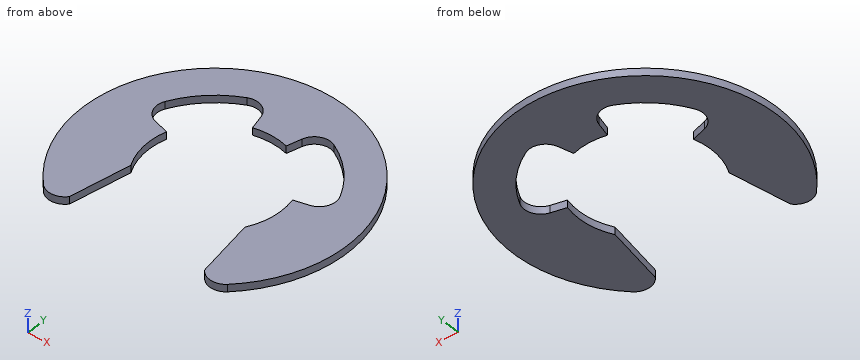
Autodesk Inventor part; units mm, degrees
ref_plane "YZ Plane" through (0, 0, 0) normal (1, 0, 0) x (0, 1, 0)
ref_plane "XZ Plane" through (0, 0, 0) normal (0, 1, 0) x (-1, 0, 0)
ref_plane "XY Plane" through (0, 0, 0) normal (0, 0, 1) x (1, 0, 0)
sketch "Sketch1" plane through (0, 0, 0) normal (0, 0, 1) x (1, 0, 0)
  arc A0 (11.7245, -15.68) -> (15.9849, -15.9849) centre (13.9867, -13.9867) ccw
  arc A1 (15.9849, -15.9849) -> (-15.9849, -15.9849) centre (0, 0) ccw
  arc A2 (-15.9849, -15.9849) -> (-11.7245, -15.68) centre (-13.9867, -13.9867) ccw
  line L0 (-11.7245, -15.68) -> (-9.8901, -5.472)
  arc A3 (-10.9218, 2.9106) -> (-9.8901, -5.472) centre (0, 0) ccw
  line L1 (-10.9218, 2.9106) -> (-13.3802, 3.5657)
  arc A4 (-15.1786, 7.5542) -> (-13.3802, 3.5657) centre (-12.6488, 6.2952) ccw
  arc A5 (-7.5542, 15.1786) -> (-15.1786, 7.5542) centre (0, 0) ccw
  arc A6 (-3.5657, 13.3802) -> (-7.5542, 15.1786) centre (-6.2952, 12.6488) ccw
  line L2 (-3.5657, 13.3802) -> (-2.9254, 10.9179)
  arc A7 (2.9254, 10.9179) -> (-2.9254, 10.9179) centre (0, 0) ccw
  line L3 (2.9254, 10.9179) -> (3.5657, 13.3802)
  arc A8 (7.5542, 15.1786) -> (3.5657, 13.3802) centre (6.2952, 12.6488) ccw
  arc A9 (15.1786, 7.5542) -> (7.5542, 15.1786) centre (0, 0) ccw
  arc A10 (13.3802, 3.5657) -> (15.1786, 7.5542) centre (12.6488, 6.2952) ccw
  line L4 (13.3802, 3.5657) -> (10.9218, 2.9106)
  arc A11 (9.8901, -5.472) -> (10.9218, 2.9106) centre (0, 0) ccw
  line L5 (9.8901, -5.472) -> (11.7245, -15.68)
  dimension "d0" = 22.606
  dimension "d2" = 11.303
extrude "Extrusion1" add sketch "Sketch1" against normal blind 1.27
properties part number "am-0206" material "Steel"
Build history of the part. All positions in model axes, mm. Coordinates: 2 decimals unless noted, no trailing zeros. Write each loop counter-clockwise with the first axis right and the second up, starting at its lowest first coordinate (ties: lowest second). Pieces come first, ordered by that corner, then holes.
(1) Drill centre lines: line 1 (X direction, y = 14, z = -0.8); line 2 (X direction, y = -6.5, z = -1.2); line 3 (Y direction, x = -15, z = -0.3). Where is each one in solid material? Low to high.
(2) Cut at B-B on z = -0.85. List the corners of the cut face in (x, y).
(3) Cut at A-A on y = 0. List the corners of the cut face in (x, z), and give its area (3 significant figures).
(4) Cut at D-D on y = 18. List the corners of the cut face in (x, z).
(5) Pin check, flat tip, straight feed: pin 1 Ø10 at (x, y) = (-3.5, -12) entering from -Z. Stop position of the tip, or through.
(6) Cut at C-C on x = 0. List the corners of the cut face in (y, z), and give its area (3 significant figures).
Working result:
1. line 1: x = -17.75 to -9.56, -3.81 to 3.81, 9.56 to 17.75
1. line 2: x = -21.65 to -10.07, 10.07 to 21.65
1. line 3: y = -16.62 to 4.73, 7.9 to 16.91
2. outline: (-15.98, -15.98) arc R2.83 ccw to (-11.72, -15.68) - (-9.89, -5.47) arc R11.3 cw to (-10.92, 2.91) - (-13.38, 3.57) arc R2.83 cw to (-15.18, 7.55) arc R16.95 cw to (-7.55, 15.18) arc R2.83 cw to (-3.57, 13.38) - (-2.93, 10.92) arc R11.3 cw to (2.93, 10.92) - (3.57, 13.38) arc R2.83 cw to (7.55, 15.18) arc R16.95 cw to (15.18, 7.55) arc R2.83 cw to (13.38, 3.57) - (10.92, 2.91) arc R11.3 cw to (9.89, -5.47) - (11.72, -15.68) arc R2.83 ccw to (15.98, -15.98) arc R22.61 ccw (long way) to start
3. outline: (-22.61, -1.27) - (-11.3, -1.27) - (-11.3, 0) - (-22.61, 0) - close; (11.3, -1.27) - (22.61, -1.27) - (22.61, 0) - (11.3, 0) - close
3. area: 28.7 mm2
4. outline: (-13.68, -1.27) - (13.68, -1.27) - (13.68, 0) - (-13.68, 0) - close
5. pin 1: passes through
6. outline: (11.3, -1.27) - (22.61, -1.27) - (22.61, 0) - (11.3, 0) - close
6. area: 14.4 mm2
